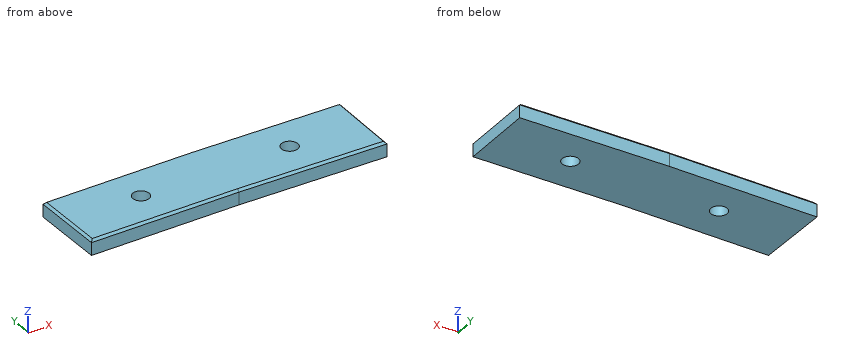
from build123d import *

# Parameters (mm, degrees)
SKETCH3_R           = 2.2
BOSS_EXTRUDE1_DEPTH = 4
CHAMFER1_SIZE       = 0.6


with BuildPart() as part:
    # Sketch3 → Boss-Extrude1 (new body)
    with BuildSketch(Plane.XY):
        Polygon((-39.988460604, 11.048492995), (-40.468829865, 31.042723297), (-0.480369261, 32.003461819), (39.51963059, 32), (39.51963059, 12), (0, 12), align=None)
        with Locations((19.759815295, 22)):
            Circle(SKETCH3_R, mode=Mode.SUBTRACT)
        with Locations((-20.234414932, 21.525977407)):
            Circle(SKETCH3_R, mode=Mode.SUBTRACT)
    extrude(amount=BOSS_EXTRUDE1_DEPTH)

    # Chamfer1
    # the kernel refuses this chamfer: 0.6 mm, written as the material it takes off along each edge
    with BuildSketch(Plane(origin=(39.51963059, 33.543009793, 4), x_dir=(0, 0, -1), z_dir=(0, -1, 0)), Plane(origin=(-39.951399881, 9.505928338, 4), x_dir=(0, 0, -1), z_dir=(-0.024018463033284497, 0.9997115151049921, 0))) as chamfer1_piece_1:
        Polygon((CHAMFER1_SIZE, 0), (0, -CHAMFER1_SIZE), (0, 0), align=None)
    extrude(amount=23.086019586, mode=Mode.SUBTRACT)
    with BuildSketch(Plane(origin=(-2.023379048, 32.003595359, 4), x_dir=(0, 0, -1), z_dir=(0.999999996254941, -8.654546850213052e-05, 0)), Plane(origin=(-42.011394523, 31.005662574, 4), x_dir=(0, 0, -1), z_dir=(0.9997115151049922, 0.02401846303328057, 0))) as chamfer1_piece_2:
        Polygon((CHAMFER1_SIZE, 0), (0, -CHAMFER1_SIZE), (0, 0), align=None)
    extrude(amount=43.086019586, mode=Mode.SUBTRACT)
    with BuildSketch(Plane(origin=(1.542573167, 12.036704818, 4), x_dir=(0, 0, -1), z_dir=(-0.9997170300986874, -0.023787806344009378, 0))) as chamfer1_piece_3_section:
        Polygon((CHAMFER1_SIZE, 0), (0, -CHAMFER1_SIZE), (0, 0), align=None)
    chamfer1_piece_3 = extrude(amount=43.085798923, mode=Mode.PRIVATE)
    chamfer1_piece_3 = split(chamfer1_piece_3, bisect_by=Plane(origin=(1.542573167, 12.318352409, 3.718352409), z_dir=(0, -0.7071067811865478, 0.7071067811865474)), keep=Keep.TOP, mode=Mode.PRIVATE)
    add(chamfer1_piece_3, mode=Mode.SUBTRACT)
    with BuildSketch(Plane(origin=(41.062640382, 12, 4), x_dir=(0, 0, -1), z_dir=(-1, 0, 0))) as chamfer1_piece_4_section:
        Polygon((CHAMFER1_SIZE, 0), (0, -CHAMFER1_SIZE), (0, 0), align=None)
    chamfer1_piece_4 = extrude(amount=42.605650175, mode=Mode.PRIVATE)
    chamfer1_piece_4 = split(chamfer1_piece_4, bisect_by=Plane(origin=(41.043886193, 12.788171977, 3.211604931), z_dir=(0.01682051917540141, -0.706906691250458, 0.7071067811865475)), keep=Keep.TOP, mode=Mode.PRIVATE)
    add(chamfer1_piece_4, mode=Mode.SUBTRACT)


solid = part.part
The model under review builds one solid part; all positions refer to its coordinate system, in mm. Give positions to 0.01 mm unless a question says otherwise; leave off trailing zeros. Loops run counter-clockwise (first coordinate to the right, second up) from the corner with the lowest first, then second, coordinate; pieces in that order, holes last. Notation, with made-up numbers: (-10, 39.25) -> (12, 39.25) arc R16 cw to (12, 70.25) -> close; hole circle Ø9 at (6, 72.25). An arc over 180 degrees is marked (long way). Put each result on its own line as item: value. Start each with the question number.
1. We need section A-A on x = -19.5. State the section outline as (y, z) points, then the cut area to 3 significant figures.
2. Wall thickness on probe 1 along X at (y, z) = (20, 2); probe 2 along Y at (x, z) = (7, 1.7); probe 3 along X at (y, z) = (15.75, 1.3): over which ranges is each line inside the solid? List them lowest first.
3. We need section B-B on z = 2.45. State the section outline as (x, y) points, then the cut area to 3 significant figures.
4. Clearance check with flat-ended pins moving along their axes: P1, Ø4, axis at x = -20.23, y = 21.53, coming from the +Z side; P2, Ø2, axis at x = -27.5, z = 1, coming from the +Y side; P3, Ø1.5, axis at y = 15.5, z = 1.5, coming from the -X side; P4, Ø2, axis at x = 12, z = 3.5, coming from the -Y side. State where each tip first meets the part, or that it passes through.
Determined:
1. outline: (11.54, 0) -> (19.45, 0) -> (19.45, 4) -> (12.14, 4) -> (11.54, 3.4) -> close; (23.6, 0) -> (31.55, 0) -> (31.55, 3.4) -> (30.95, 4) -> (23.6, 4) -> close
1. area: 63.1 mm^2
2. probe 1: -40.2 to -21.82, -18.65 to 18.84, 20.68 to 39.52
2. probe 2: 12 to 32
2. probe 3: -40.1 to 39.52
3. outline: (-40.47, 31.04) -> (-39.99, 11.05) -> (0, 12) -> (39.52, 12) -> (39.52, 32) -> (-0.48, 32) -> close; hole circle Ø4.4 at (-20.23, 21.53); hole circle Ø4.4 at (19.76, 22)
3. area: 1,570 mm^2
4. P1: through
4. P2: y = 31.38
4. P3: x = -40.11
4. P4: y = 12
